```python
from build123d import *

# Parameters (mm, degrees)
F1_DEPTH = 1
F2_DEPTH = 40
F3_R     = 0.5


with BuildPart() as f1:
    # F0 (on Front) → F1 (new body)
    with BuildSketch(Plane.XZ):
        with BuildLine():
            ThreePointArc((-7.75, 0), (-2.269922, 2.269922), (0, 7.75))
            Line((0, 7.75), (0, 23.041173))
            ThreePointArc((0, 23.041173), (-2.679639, 28.902397), (-8.865534, 30.710468))
            Line((-8.865534, 30.710468), (-49.863639, 24.747107))
            ThreePointArc((-49.863639, 24.747107), (-53.537722, 22.735029), (-55, 18.809588))
            Line((-55, 18.809588), (-55, 6))
            ThreePointArc((-55, 6), (-53.242641, 1.757359), (-49, 0))
            Line((-49, 0), (-7.75, 0))
        make_face()
    extrude(amount=F1_DEPTH)

    # F0 (on Front) → F2 (join)
    with BuildSketch(Plane.XZ):
        with BuildLine():
            Line((-49, -1.6), (-7.75, -1.6))
            ThreePointArc((-7.75, -1.6), (-1.138552, 1.138552), (1.6, 7.75))
            Line((1.6, 7.75), (1.6, 23.041173))
            ThreePointArc((1.6, 23.041173), (-1.632855, 30.112456), (-9.095838, 32.293806))
            Line((-9.095838, 32.293806), (-50.093943, 26.330445))
            ThreePointArc((-50.093943, 26.330445), (-54.747781, 23.781813), (-56.6, 18.809588))
            Line((-56.6, 18.809588), (-56.6, 6))
            ThreePointArc((-56.6, 6), (-54.374012, 0.625988), (-49, -1.6))
        make_face()
        with BuildLine():
            Line((0, 23.041173), (0, 7.75))
            ThreePointArc((0, 7.75), (-2.269922, 2.269922), (-7.75, 0))
            Line((-7.75, 0), (-49, 0))
            ThreePointArc((-49, 0), (-53.242641, 1.757359), (-55, 6))
            Line((-55, 6), (-55, 18.809588))
            ThreePointArc((-55, 18.809588), (-53.537722, 22.735029), (-49.863639, 24.747107))
            Line((-49.863639, 24.747107), (-8.865534, 30.710468))
            ThreePointArc((-8.865534, 30.710468), (-2.679639, 28.902397), (0, 23.041173))
        make_face(mode=Mode.SUBTRACT)
    extrude(amount=F2_DEPTH)

    # F3
    f3_edges = [f1.edges().sort_by_distance(p)[0] for p in [
        (-29.59489, -40, 29.312126),
        (-29.364586, -40, 27.728787),
    ]]
    fillet(f3_edges, radius=F3_R)


solid = f1.part
```
Verification items for the finished model (mm, model axes). A direction names the side the tool comes from. Round coordinates to 2 decimals unless told otherwise and drop trailing zeros. Write each loop counter-clockwise with the first axis right and the second up, starting at its lowest first coordinate (ties: lowest second). Pieces come first, ordered by that corner, then holes. Notation, with made-up numbers: (-10, 55) -> (14, 55) arc R34 ccw to (14, 93) -> close; hole circle Ø7 at (64.25, -38). An arc over 180 degrees is marked (long way). Write each question's results on one line, items separated by ' | '.
Q1. Go/stop test with flat-tipped pins: pin 1 Ø2 at (y, z) = (-30, 21.5) entering from -X; pin 2 Ø3 at (x, y) = (-48, -26) entering from +Z; pin 3 Ø5 at (x, z) = (-20.5, 15.5) entering from -Y. Record where each tip stops, or that it passes through.
Derived:
pin 1: stops at x = -56.41 | pin 2: stops at z = 26.85 | pin 3: stops at y = -1
Q2. Sectioned sample at B-B, the plane z = 8.5. Record the boundary of the cut face in (x, y).
Derived:
outline: (-56.6, -39.5) arc R0.5 ccw to (-56.1, -40) -> (-55.5, -40) arc R0.5 ccw to (-55, -39.5) -> (-55, -1) -> (0, -1) -> (0, -39.5) arc R0.5 ccw to (0.5, -40) -> (1.1, -40) arc R0.5 ccw to (1.6, -39.5) -> (1.6, 0) -> (-56.6, 0) -> close
Q3. Sectioned sample at A-A, the plane y = -11. Record the boundary of the cut face in (x, z).
Derived:
outline: (-56.6, 6) arc R7.6 ccw to (-49, -1.6) -> (-7.75, -1.6) arc R9.35 ccw to (1.6, 7.75) -> (1.6, 23.04) arc R9.35 ccw to (-9.1, 32.29) -> (-50.09, 26.33) arc R7.6 ccw to (-56.6, 18.81) -> close; hole (-55, 6) arc R6 ccw to (-49, 0) -> (-7.75, 0) arc R7.75 ccw to (0, 7.75) -> (0, 23.04) arc R7.75 ccw to (-8.87, 30.71) -> (-49.86, 24.75) arc R6 ccw to (-55, 18.81) -> close
Q4. Draft check along Z on faces 1 (the face through (-2.21, -19.98, 2.33)), 2 (the face through (-29, -19, -1.6)), 3 (the face through (-56.6, -19, 12)). Enter one of: released by +Z, released by -Z, zero draft, split by the parting line, or undercut.
Derived:
face 1: undercut | face 2: released by -Z | face 3: zero draft
Q5. Thickness scan on probe 1 along X at (y, z) = (-9, 12); probe 2 along Y at (x, z) = (-20, 1.5); probe 3 along X at (y, z) = (-20.5, 20). Record the ranges inside material, lowest first.
Derived:
probe 1: x = -56.6 to -55, 0 to 1.6 | probe 2: y = -1 to 0 | probe 3: x = -56.51 to -54.88, 0 to 1.6
Q6. Access from +Z, -Z, +X, -X, +Y, -Y to the whole of each face (thin tool, end or side, straight path). Record for faces 4 (the face through (-29.308, -19.474, 29.354)), 5 (the face through (-28, -20, 0)).
Derived:
face 4: +Z, -X, +Y, -Y | face 5: -Y
